Design review of the part built by this model. Coordinates are the model's own, in mm. Face numbers are marked on the shaded views. A direction names the side the tool comes from. Give positions to 0.01 mm unless a question says otherwise; leave off trailing zeros. Write each loop counter-clockwise with the first axis right and the second up, starting at its lowest first coordinate (ties: lowest second). Pieces come first, ordered by that corner, then holes. Notation, with made-up numbers: (3, 39.25) -> (45, 39.25) arc R17 cw to (45, 47.25) -> close; hole circle Ø6 at (-14.75, 15). An arc over 180 degrees is marked (long way). Answer as a JSON object with one key per item and string values.
```python
from build123d import *

# Parameters (mm, degrees)
F0_W      = 42.418
F0_H      = 42.418
F1_DEPTH  = 10
F2_SIZE   = 7.62
F4_DEPTH  = 10
F5_SIZE   = 5.08
F7_DEPTH  = 10
F8_R      = 10.9982
F9_DEPTH  = 2
F10_R     = 2.5
F11_DEPTH = 22
F13_DEPTH = 15
F14_R     = 1.5
F15_DEPTH = 6.35


with BuildPart() as f1:
    # F0 (on Top) → F1 (new body, symmetric)
    with BuildSketch(Plane.XY):
        Rectangle(F0_W, F0_H)
    extrude(amount=F1_DEPTH, both=True)

    # F2
    f2_edges = [f1.edges().sort_by_distance(p)[0] for p in [
        (21.209, 21.209, 0),
        (-21.209, 21.209, 0),
        (-21.209, -21.209, 0),
        (21.209, -21.209, 0),
    ]]
    chamfer(f2_edges, length=F2_SIZE)

    # F3 (on face) → F4 (join)
    with BuildSketch(Plane.XY.offset(10)):
        Polygon((13.589, 21.209), (-13.589, 21.209), (-21.209, 13.589), (-21.209, -13.589), (-13.589, -21.209), (13.589, -21.209), (21.209, -13.589), (21.209, 13.589), align=None)
        Polygon((21.209, 21.209), (13.589, 21.209), (21.209, 13.589), align=None)
        Polygon((-13.589, 21.209), (-21.209, 21.209), (-21.209, 13.589), align=None)
        Polygon((-13.589, -21.209), (-21.209, -13.589), (-21.209, -21.209), align=None)
        Polygon((21.209, -21.209), (21.209, -13.589), (13.589, -21.209), align=None)
    extrude(amount=F4_DEPTH)

    # F5
    f5_edges = [f1.edges().sort_by_distance(p)[0] for p in [
        (21.209, 21.209, 15),
        (-21.209, 21.209, 15),
        (-21.209, -21.209, 15),
        (21.209, -21.209, 15),
    ]]
    chamfer(f5_edges, length=F5_SIZE)

    # F6 (on face) → F7 (join)
    with BuildSketch(Plane(origin=(0, 0, -10), x_dir=(1, 0, 0), z_dir=(0, 0, -1))):
        Polygon((-13.589, 21.209), (-16.129, 21.209), (-21.209, 16.129), (-21.209, 13.589), align=None)
        Polygon((16.129, 21.209), (13.589, 21.209), (21.209, 13.589), (21.209, 16.129), align=None)
        Polygon((21.209, -16.129), (21.209, -13.589), (13.589, -21.209), (16.129, -21.209), align=None)
        Polygon((-13.589, -21.209), (-21.209, -13.589), (-21.209, -16.129), (-16.129, -21.209), align=None)
        Polygon((13.589, 21.209), (-13.589, 21.209), (-21.209, 13.589), (-21.209, -13.589), (-13.589, -21.209), (13.589, -21.209), (21.209, -13.589), (21.209, 13.589), align=None)
    extrude(amount=F7_DEPTH)

    # F8 (on face) → F9 (join)
    with BuildSketch(Plane.XY.offset(20)):
        Circle(F8_R)
    extrude(amount=F9_DEPTH)

    # F10 (on face) → F11 (join)
    with BuildSketch(Plane.XY.offset(22)):
        Circle(F10_R)
    extrude(amount=F11_DEPTH)

    # F12 (on face) → F13 (cut)
    with BuildSketch(Plane.XY.offset(44)):
        with BuildLine():
            Line((2.6203631624, 2.9334036984), (-2.6333660554, 2.9334036984))
            Line((-2.6333660554, 2.9334036984), (-2.6333660554, 2))
            Line((-2.6333660554, 2), (-1.5, 2))
            ThreePointArc((-1.5, 2), (0, 2.5), (1.5, 2))
            Line((1.5, 2), (2.6203631624, 2))
            Line((2.6203631624, 2), (2.6203631624, 2.9334036984))
        make_face()
        with BuildLine():
            ThreePointArc((1.5, 2), (0, 2.5), (-1.5, 2))
            Line((-1.5, 2), (1.5, 2))
        make_face()
    extrude(amount=-F13_DEPTH, mode=Mode.SUBTRACT)

    # F14 (on face) → F15 (cut)
    with BuildSketch(Plane.XY.offset(20)):
        with Locations((-15.5, 15.5)):
            Circle(F14_R)
        with Locations((15.5, 15.5)):
            Circle(F14_R)
        with Locations((15.5, -15.5)):
            Circle(F14_R)
        with Locations((-15.5, -15.5)):
            Circle(F14_R)
    extrude(amount=-F15_DEPTH, mode=Mode.SUBTRACT)


with BuildPart() as f16_1:
    # F16: copy of F1
    add(f1.part)


solid = f1.part
```
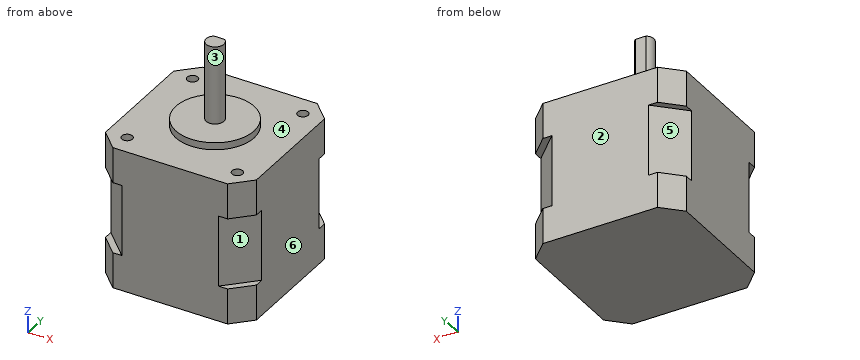
(1) We need section D-D, the plane x = 9. State the section outline as (y, z) points.
Here are the results:
{"outline": "(-21.21, -20) -> (21.21, -20) -> (21.21, 20) -> (6.32, 20) -> (6.32, 22) -> (-6.32, 22) -> (-6.32, 20) -> (-21.21, 20) -> close"}
(2) We need section C-C, the plane x = 0. State the section outline as (y, z) points, then the cut area to 3 significant figures.
Here are the results:
{"outline": "(-21.21, -20) -> (21.21, -20) -> (21.21, 20) -> (11, 20) -> (11, 22) -> (2.5, 22) -> (2.5, 29) -> (2, 29) -> (2, 44) -> (-2.5, 44) -> (-2.5, 22) -> (-11, 22) -> (-11, 20) -> (-21.21, 20) -> close", "area": "1,840 mm²"}
(3) Clearance check with flat-ended pins moving along their axes: pin 1 (10 mm diameter, centred on x = -6, z = 26, fed in from +Y); pin 2 (8.5 mm diameter, centred on x = 16, y = 17, fed in from +Z); pin 3 (6 mm diameter, centred on y = 6.5, z = 32, fed in from +X); pin 4 (0.9 mm diameter, centred on x = 0, z = 34.5, fed in from +Y). State where each tip first meets the part, or that it passes through.
Here are the results:
{"pin 1": "stops at y = 10.58", "pin 2": "stops at z = 20", "pin 3": "passes through", "pin 4": "stops at y = 2"}
(4) For the marked faces 1, 2 and 3, list the 3-axis set-ups (+Z, -Z, +X, -X, +Y, -Y) from which the entire face can be reached by the end or side of a thin tool; tool diameter is ignored.
Here are the results:
{"face 1": "+X, -Y", "face 2": "+Z, -Z, +X, -X, +Y", "face 3": "+Z"}
(5) We need section A-A, the plane y = 0. State the section outline as (x, z) points.
Here are the results:
{"outline": "(-21.21, -20) -> (21.21, -20) -> (21.21, 20) -> (11, 20) -> (11, 22) -> (2.5, 22) -> (2.5, 44) -> (-2.5, 44) -> (-2.5, 22) -> (-11, 22) -> (-11, 20) -> (-21.21, 20) -> close"}
(6) The part is to be moulded in two halves that separate along Z. For the marked faces 4, 5 and 6, say which applies: +Z half, -Z half, draft (parallel to the pull), parting line (faces both ways), or undercut.
Here are the results:
{"face 4": "+Z half", "face 5": "undercut", "face 6": "draft"}
(7) We need section B-B, the plane z = 4.5. State the section outline as (x, y) points, then the cut area to 3 significant figures.
Here are the results:
{"outline": "(-21.21, -13.59) -> (-13.59, -21.21) -> (13.59, -21.21) -> (21.21, -13.59) -> (21.21, 13.59) -> (13.59, 21.21) -> (-13.59, 21.21) -> (-21.21, 13.59) -> close", "area": "1,680 mm²"}
(8) For line 1 along Y through (x, z) = (15.5, 18); line 2 along X through (y, z) = (-15, 18); line 3 along Z through (x, y) = (-6.5, -2), list the stretches that pass through material, from the lowest coordinate up.
Here are the results:
{"line 1": "y = -21.21 to -17, -14 to 14, 17 to 21.21", "line 2": "x = -21.21 to -16.91, -14.09 to 14.09, 16.91 to 21.21", "line 3": "z = -20 to 22"}
